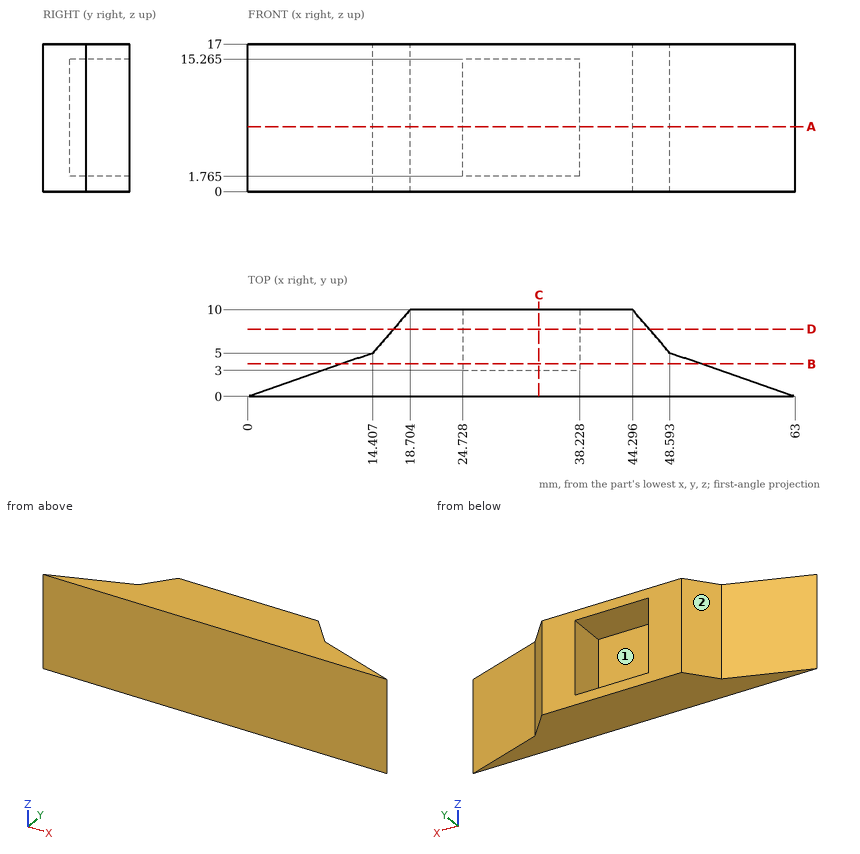
Source: three-view drawing plus pictorial views. Frame: mm from the lowest corner of the part. A direction names the side the tool comes from. Give positions to 0.01 mm unless a question says otherwise; leave off trailing zeros. Order: outer loops, then holes, each group sorted by start corner. A loop starts at its lowest first (then second) coordinate and runs counter-clockwise, first axis right, second up. Notation, with made-up numbers: M 21,-10.75 L 59,-10.75 A13 ccw 59,13.25 Z; hole C -29,-23.75 d11. An arc over 180 degrees is marked long. One line per question, with ' | ' between items.
1) Section D-D on y = 7.75. Output: boundary loops of the cut face in (x, z) (1 decimal).
Filled in:
outline: M 16.8,0 L 46.2,0 L 46.2,17 L 16.8,17 Z; hole M 24.7,1.8 L 38.2,1.8 L 38.2,15.3 L 24.7,15.3 Z
2) Access query for the marked faces 1 and 2. Directions: +Z, -Z, +X, -X, +Y, -Y. A direction counts if a zero-diameter tool reaches every point of the face in a straight line with its end or side. Return the directions, or none.
Filled in:
face 1: +Y | face 2: +Z, -Z, -X, +Y
3) Section B-B on y = 3.75. Output: boundary loops of the cut face in (x, z) (1 decimal).
Filled in:
outline: M 10.8,0 L 52.2,0 L 52.2,17 L 10.8,17 Z; hole M 24.7,1.8 L 38.2,1.8 L 38.2,15.3 L 24.7,15.3 Z
4) Ray query, L1, parallel to Z at x = 29, y = 6 (1 decimal); L2, parallel to Y at x = 33.5, z = 5; L3, parallel to X at y = 9.25, z = 7.5. Return the intervals inside material, ascending.
Filled in:
L1: z = 0 to 1.8, 15.3 to 17 | L2: y = 0 to 3 | L3: x = 18.06 to 24.73, 38.23 to 44.94
5) Contact query for flat-ended pins moving along their axis: P1, Ø3.5, axis at y = 7, z = 5.5, coming from the -X side; P2, Ø7, axis at x = 32.5, z = 6, coming from the +Y side. Output: stop coordinate, or through.
Filled in:
P1: stops at x = 14.62 | P2: stops at y = 3
6) Section C-C on x = 33.5. Output: boundary loops of the cut face in (y, z) (1 decimal).
Filled in:
outline: M 0,0 L 10,0 L 10,1.8 L 3,1.8 L 3,15.3 L 10,15.3 L 10,17 L 0,17 Z
7) Section A-A on z = 7.5. Output: boundary loops of the cut face in (x, y) (1 decimal).
Filled in:
outline: M 0,0 L 63,0 L 48.6,5 L 44.3,10 L 38.2,10 L 38.2,3 L 24.7,3 L 24.7,10 L 18.7,10 L 14.4,5 Z
